Can you work these out from the model? Positions are in its coordinate system, mm. A direction names the side the tool comes from. Round coordinates to 2 decimals unless told otherwise and drop trailing zeros. Write each loop counter-clockwise with the first axis right and the second up, starting at its lowest first coordinate (ties: lowest second). Pieces come first, ordered by that corner, then holes.
Q1. For faces 1 (the cylindrical face through (5.744, 69.857, 0.601)), 2 (the conical face through (14.008, 16.768, 2.344)), 3 (the cylindrical face through (15.23, 19.88, 8.46)), 4 (the flat face through (-22, 51, 4)), 5 (the cylindrical face through (-24.59, 51.89, 3.97)), which set-ups out of +Z, -Z, +X, -X, +Y, -Y let a thin tool reach every point of the face, with its end or its side?
Q2. I'm going to push flat-ended pins straight in: pin 1 Ø1.5 at (y, z) = (66, 5.5) entering from -X; pin 2 Ø6 at (y, z) = (42.5, 1.5) entering from +X; pin 3 Ø5 at (x, z) = (-13.5, 6.5) entering from -Y; pin 4 Ø6 at (x, z) = (3.5, 7) entering from -Y. Where does each tip first touch, or does it pass through?
Q3. We'd pull the mould along X, two halves only. Please class faces 6 (the cylindrical face through (5.957, 37.273, 7.184)), 7 (the cylindrical face through (26.25, 37.22, 3.97)), 8 (the flat face through (5, 37, 12)): +X half, -X half, draft (parallel to the pull), parting line (faces both ways), or undercut.
Q4. Please list where these lines run through material, in increasing order: line 1 along Z through (x, y) = (-0.5, 39.5); line 2 along Y through (x, z) = (5, 9.75); line 3 along X through (y, z) = (43, 10.5).
Q5. If we section it at A-A (z = 9): Please give me the cut outline in (x, y).
Q6. If we section it at B-B (z = 3.75): Please give me the cut outline in (x, y), plus the area to 3 significant figures.
Autodesk Inventor part; units mm, degrees
ref_plane "YZ Plane" through (0, 0, 0) normal (1, 0, 0) x (0, 1, 0)
ref_plane "XZ Plane" through (0, 0, 0) normal (0, 1, 0) x (-1, 0, 0)
ref_plane "XY Plane" through (0, 0, 0) normal (0, 0, 1) x (1, 0, 0)
sketch "Sketch1" plane through (0, 0, 0) normal (0, 0, 1) x (1, 0, 0)
  arc A0 (4.1897, 73.9335) -> (-24.7532, 53.8125) centre (6.3147, 40) ccw
  arc A1 (-24.7532, 53.8125) -> (-22.9256, 51) centre (-22.9256, 53) ccw
  line L0 (-22.9256, 51) -> (-20.5538, 51)
  arc A2 (-11.7644, 45.7692) -> (-20.5538, 51) centre (-20.5538, 41) ccw
  arc A3 (-2.9879, 3.2692) -> (-11.7644, 45.7692) centre (-77.6853, 10) ccw
  arc A4 (-2.9879, 3.2692) -> (0, 0) centre (0, 3) ccw
  line L1 (0, 0) -> (33.3057, 0)
  arc A5 (33.3057, 0) -> (36.2787, 3.4018) centre (33.3057, 3) ccw
  arc A6 (36.2787, 3.4018) -> (7.1029, 65.6915) centre (-77.6853, -12) ccw
  arc A7 (6.3147, 67.7183) -> (7.1029, 65.6915) centre (9.3147, 67.7183) ccw
  line L2 (6.3147, 67.7183) -> (6.3147, 71.9374)
  arc A8 (6.3147, 71.9374) -> (4.1897, 73.9335) centre (4.3147, 71.9374) ccw
  circle A9 centre (6.3147, 40) radius 2.75
  circle A10 centre (16.3147, 15) radius 2.75
extrude "Extrusion1" add sketch "Sketch1" along normal blind 6
fillet "Fillet1" radius 2 12 edges at (26.457, 36.7791, 0) (6.5187, 66.631, 0) (6.3147, 69.8278, 0) (5.684, 73.3952, 0) (-13.0929, 67.9167, 0) (-24.6027, 51.9103, 0) (-21.7397, 51, 0) (-15.4398, 49.5934, 0) (-4.235, 25.1679, 0) (-2.2145, 0.9761, 0) (16.6529, 0, 0) (35.5646, 1.0258, 0)
chamfer "Chamfer1" distance 2.5 angle 45 1 edges at (3.5647, 40, 0)
chamfer "Chamfer2" distance 2.5 angle 45 1 edges at (13.5647, 15, 0)
sketch "Sketch2" plane through (0, 0, 6) normal (0, 0, 1) x (1, 0, 0)
  circle A0 centre (6.3147, 40) radius 2.75
  circle A1 centre (16.3147, 15) radius 2.75
  circle A2 centre (6.3147, 40) radius 5
  circle A3 centre (16.3147, 15) radius 5
  point P0 (0, 0)
extrude "Extrusion2" add sketch "Sketch2" along normal blind 6
chamfer "Chamfer3" distance 1 angle 45 1 edges at (1.3147, 40, 12)
chamfer "Chamfer4" distance 1 angle 45 1 edges at (11.3147, 15, 12)
properties part number "Rukohvat_Desni_4"
A:
1. face 1: -Z, +X, +Y
1. face 2: -Z
1. face 3: +Z
1. face 4: +Z, -Z, -X, -Y
1. face 5: +Z, -Z, -X
2. pin 1: stops at x = -16.45
2. pin 2: stops at x = 25.12
2. pin 3: stops at y = 44.42
2. pin 4: stops at y = 0
3. face 6: undercut
3. face 7: +X half
3. face 8: draft
4. line 1: z = 0 to 6
4. line 2: y = 35.18 to 37.58, 42.42 to 44.82
4. line 3: x = 2.31 to 10.31
5. outline: circle Ø10 at (6.31, 40); circle Ø10 at (16.31, 15); hole circle Ø5.5 at (6.31, 40); hole circle Ø5.5 at (16.31, 15)
6. outline: (-24.75, 53.81) arc R2 ccw to (-22.93, 51) - (-20.55, 51) arc R10 cw to (-11.76, 45.77) arc R75 cw to (-2.99, 3.27) arc R3 ccw to (0, 0) - (33.31, 0) arc R3 ccw to (36.28, 3.4) arc R115 ccw to (7.1, 65.69) arc R3 cw to (6.31, 67.72) - (6.31, 71.94) arc R2 ccw to (4.19, 73.93) arc R34 ccw to start; hole circle Ø5.5 at (6.31, 40); hole circle Ø5.5 at (16.31, 15)
6. area: 2,420 mm2
